Geometry: final body of the model. Coordinates: model frame, mm. Coordinates: 2 decimals unless noted, no trailing zeros. Order: outer loops, then holes, each group sorted by start corner. A loop starts at its lowest first (then second) coordinate and runs counter-clockwise, first axis right, second up. Notation, with made-up numbers: (73.25, 87.5) - (110.25, 87.5) arc R12 ccw to (110.25, 91.5) - close; hole circle Ø4 at (14, 53.25). An arc over 180 degrees is marked (long way). Use one line per item in the form item = value. Start each with the question number.
```python
from build123d import *

# Parameters (mm, degrees)
SKETCH1_W           = 38.1
SKETCH1_H           = 38.1
BOSS_EXTRUDE1_DEPTH = 12.7
CUT_EXTRUDE1_REACH  = 14.7
SKETCH2_R           = 5.588


with BuildPart() as part:
    # Sketch1 → Boss-Extrude1 (new body)
    with BuildSketch(Plane(origin=(0, 0, 0), x_dir=(1, 0, 0), z_dir=(0, 1, 0))):
        Rectangle(SKETCH1_W, SKETCH1_H)
    extrude(amount=BOSS_EXTRUDE1_DEPTH)

    # Sketch2 → Cut-Extrude1 (cut, up to next)
    with BuildSketch(Plane(origin=(0, 12.7, 0), x_dir=(1, 0, 0), z_dir=(0, 1, 0)), mode=Mode.PRIVATE) as cut_extrude1_sk1:
        Circle(SKETCH2_R)
    cut_extrude1_tool1 = extrude(cut_extrude1_sk1.sketch, amount=-CUT_EXTRUDE1_REACH, mode=Mode.PRIVATE) & part.part
    add(cut_extrude1_tool1.solids().sort_by_distance((0, 12.7, 0))[0], mode=Mode.SUBTRACT)


solid = part.part
```
(1) Cut plane C-C on y = 6.25. Return the cut outline in (x, z), plus the area to 3 significant figures.
(2) Cut plane B-B on x = 0. Return the cut outline in (y, z).
(3) Material intervals for L1, parallel to X at y = 9.25, z = 0; L2, parallel to X at y = 11.75, z = 5, sorted ascending. Write a range as from..to.
(4) Draft query along X for faces 1 (the flat face through (19.05, 6, 0)), 2 (the cylindrical face through (-4.434, 6.439, 3.4)), 3 (the flat face through (-19.05, 6, 0)). Return one class per face: released by +X, released by -X, zero draft, split by the parting line, or undercut.
(5) Cut plane A-A on z = 0. Return the cut outline in (x, y).
Check sheet entries:
q1.outline = (-19.05, -19.05) - (19.05, -19.05) - (19.05, 19.05) - (-19.05, 19.05) - close; hole circle Ø11.18 at (0, 0)
q1.area = 1,350 mm^2
q2.outline = (0, -19.05) - (12.7, -19.05) - (12.7, -5.59) - (0, -5.59) - close; (0, 5.59) - (12.7, 5.59) - (12.7, 19.05) - (0, 19.05) - close
q3.L1 = -19.05..-5.59, 5.59..19.05
q3.L2 = -19.05..-2.5, 2.5..19.05
q4.face_1 = released by +X
q4.face_2 = undercut
q4.face_3 = released by -X
q5.outline = (-19.05, 0) - (-5.59, 0) - (-5.59, 12.7) - (-19.05, 12.7) - close; (5.59, 0) - (19.05, 0) - (19.05, 12.7) - (5.59, 12.7) - close
